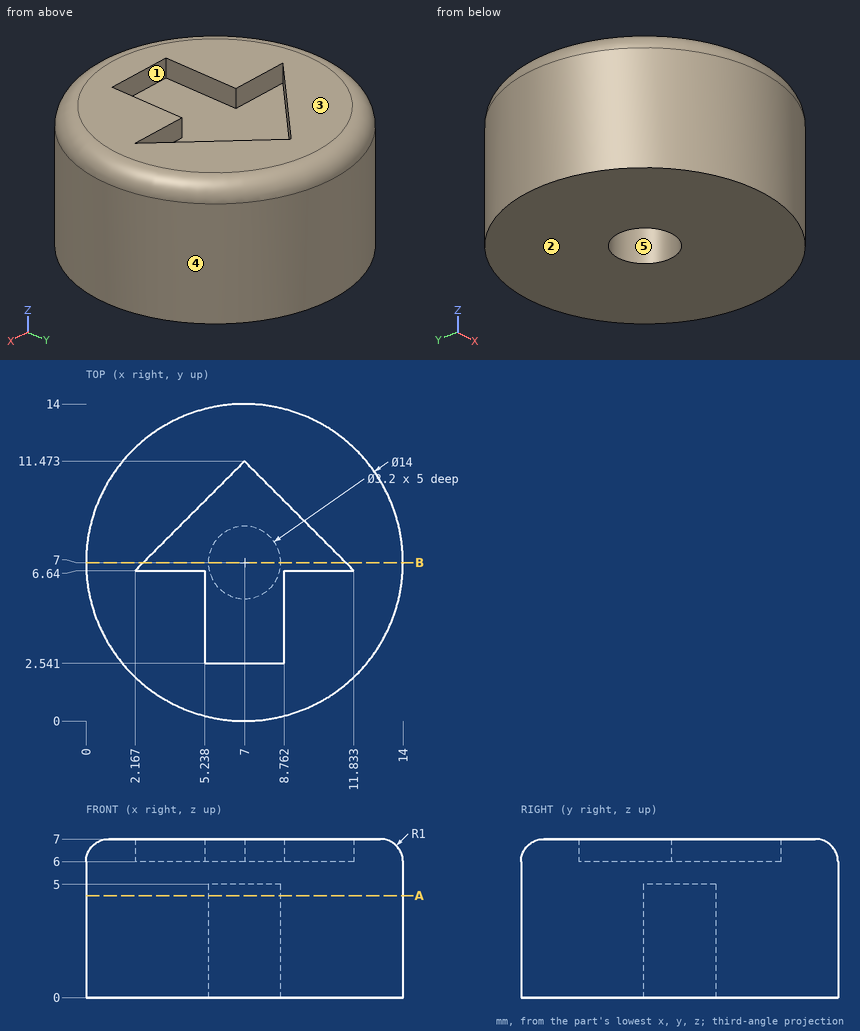
Design review of the part shown in the three views and the two pictorial views. Dimensions are in mm from the part's minimum x, y and z. A direction names the side the tool comes from. Give positions to 0.01 mm unless a question says otherwise; leave off trailing zeros. Loops run counter-clockwise (first coordinate to the right, second up) from the corner with the lowest first, then second, coordinate; pieces in that order, holes last. Notation, with made-up numbers: (10.5, -32.5) -> (17.5, -32.5) arc R22 ccw to (17.5, 3.5) -> close; hole circle Ø1 at (85.5, 12). An arc over 180 degrees is marked (long way). One line per item, written item: value.
Q1. Machinability: for the marked faces 1 and 2, which of the approach directions +Z, -Z, +X, -X, +Y, -Y give a long, thin tool a straight path to every point of the face, cutting with its end or side? Answer none if there is none.
Numbers:
face 1: +Z
face 2: -Z, +X, -X, +Y, -Y
Q2. For pin 1 Ø1.1 at (x, z) = (9.5, 6.5) entering from +Y (1 decimal); pin 2 Ø4 at (y, z) = (2, 4.5) entering from +X (1 decimal); pin 3 Ø3 at (x, y) = (7, 7) entering from -Z, all flat-tipped, find the tip position at first contact; note any pin that passes through.
Numbers:
pin 1: stops at y = 13.7
pin 2: stops at x = 13.3
pin 3: stops at z = 5
Q3. Draft analysis for pull direction X (two halves, no side actions). For the marked faces 3, 4 and 5, state which applies: pulls with the +X half, pulls with the -X half, needs draft (parallel to the pull), parting line crosses it, or undercut.
Numbers:
face 3: needs draft
face 4: parting line crosses it
face 5: undercut
Q4. For L1, parallel to Y at x = 7, z = 3.25; L2, parallel to Z at x = 1, y = 6.25; L3, parallel to Z at x = 8, y = 4.25, list the stretches that pass through material, from the lowest coordinate up.
Numbers:
L1: y = 0 to 5.4, 8.6 to 14
L2: z = 0 to 7
L3: z = 0 to 6
Q5. We need section A-A on z = 4.5. Give the boundary of the cut face in (x, y), and give its area (3 significant figures).
Numbers:
outline: circle Ø14 at (7, 7); hole circle Ø3.2 at (7, 7)
area: 146 mm^2
Q6. We need section B-B on y = 7. Give the boundary of the cut face in (x, z).
Numbers:
outline: (0, 0) -> (5.4, 0) -> (5.4, 5) -> (8.6, 5) -> (8.6, 0) -> (14, 0) -> (14, 6) arc R1 ccw to (13, 7) -> (11.47, 7) -> (11.47, 6) -> (2.53, 6) -> (2.53, 7) -> (1, 7) arc R1 ccw to (0, 6) -> close
